For this review, take the finished solid that the model builds, in its own axes (mm). A direction names the side the tool comes from. Give positions to 0.01 mm unless a question says otherwise; leave off trailing zeros. Write each loop counter-clockwise with the first axis right and the second up, starting at its lowest first coordinate (ties: lowest second). Pieces come first, ordered by that corner, then holes. Notation, with made-up numbers: M -29.5,15 L 19.5,15 A5 ccw 19.5,19 Z; hole C 17.25,54.25 d3. An arc over 180 degrees is marked long. One line per item, written item: value. Start each with the question number.
Item 1: Consider section B-B, the plane y = -9. Write out the cut boundary in (x, z), and give its area (3 significant figures).
Item 2: Tool access review of faces 4 (the face through (1.426, -20.855, 23.462)), 5 (the face through (14.79, 1.06, 20.25)), 6 (the face through (28.496, -20.855, 23.54)): name each direction out of +Z, -Z, +X, -X, +Y, -Y from which nothing blocks a thin tool from reaching the whole face with its end or side.
Item 3: Consider section C-C, the plane z = 26.5. Write out the cut boundary in (x, y), and give its area (3 significant figures).
Item 4: Clearance check with flat-ended pins moving along their axes: pin 1 Ø6 at (x, y) = (8, -7.5) entering from +Z; pin 2 Ø1.3 at (x, y) = (17.5, -20.5) entering from +Z. State where each tip first meets the part, or that it passes through.
Item 5: Consider section A-A, the plane x = 23.25. Write out the cut boundary in (y, z).
Item 6: To check wall thickness, follow probe 1 along Y at (x, z) = (22.75, 17.5); probe 2 along Y at (x, z) = (26, 11); probe 3 along Z at (x, y) = (19, -16). State the ranges of each line that lie inside material, in increasing order.
Item 7: Mouldability with a two-part tool opening along Y and no side actions: class faces 1 (the face through (15, -45.058, -48)), 2 (the face through (15, -21, 24.966)), 3 (the face through (14.79, -19.355, 12.308)) as released by +Y, released by -Y, zero draft, split by the parting line, or undercut.
```python
from build123d import *

# Parameters (mm, degrees)
F1_DEPTH = 30
F2_R     = 22.1
F3_R     = 5


with BuildPart() as f1:
    # F0 (on Right) → F1 (new body)
    with BuildSketch(Plane.YZ):
        Polygon((2.0934382497, 39.9451813902), (0, 0), (-20, 0), (-18.6916010939, 24.9657383689), (-45.0580844926, 24.9657383689), (-45.0580844926, -100.0548186098), (64.9419155074, -100.0548186098), (64.9419155074, 39.9451813902), align=None)
    extrude(amount=F1_DEPTH)

    # F2
    f2_edges = [f1.edges().sort_by_distance(p)[0] for p in [
        (15, -45.058084, 24.965738),
    ]]
    fillet(f2_edges, radius=F2_R)

    # F3
    f3_edges = [f1.edges().sort_by_distance(p)[0] for p in [
        (30, -38.585144, 18.492798),
        (0, -38.585144, 18.492798),
        (30, -20.824843, 24.965738),
        (0, -20.824843, 24.965738),
    ]]
    fillet(f3_edges, radius=F3_R)


solid = f1.part
```
Model answer:
1. outline: M 0,-100.05 L 30,-100.05 L 30,0 L 0,0 Z
1. area: 3,000 mm2
2. face 4: +Z, -X, -Y
2. face 5: +Z, +X, -X
2. face 6: +Z, +X, -Y
3. outline: M 0,1.39 L 30,1.39 L 30,64.94 L 0,64.94 Z
3. area: 1,910 mm2
4. pin 1: stops at z = 0
4. pin 2: stops at z = 24.97
5. outline: M -45.06,-100.05 L 64.94,-100.05 L 64.94,39.95 L 2.09,39.95 L 0,0 L -20,0 L -18.69,24.97 L -22.96,24.97 A22.1 ccw -45.06,2.87 Z
6. probe 1: y = -39.52 to -19.08, 0.92 to 64.94
6. probe 2: y = -43.4 to -19.42, 0.58 to 64.94
6. probe 3: z = -100.05 to 0
7. face 1: released by -Y
7. face 2: zero draft
7. face 3: undercut
